Geometry: final body of the model. Coordinates: model frame, mm. A direction names the side the tool comes from. Give positions to 0.01 mm unless a question says otherwise; leave off trailing zeros. Write each loop counter-clockwise with the first axis right and the second up, starting at its lowest first coordinate (ties: lowest second). Pieces come first, ordered by that corner, then holes.
from build123d import *

# Parameters (mm, degrees)
BOSS_EXTRUDE1_DEPTH      = 280
BOSS_EXTRUDE1_DEPTH_BACK = 20


with BuildPart() as part:
    # Sketch1 → Boss-Extrude1 (new, two sides: drawn at the far end of the back side and taken through both)
    with BuildSketch(Plane.XY.offset(-BOSS_EXTRUDE1_DEPTH_BACK)):
        with BuildLine():
            Line((-170.37773053, -331.05), (-168.636, -331.05))
            Line((-168.636, -331.05), (-168.636, -59.198829312))
            ThreePointArc((-168.636, -59.198829312), (-165.748851618, -48.847485946), (-157.920969051, -41.484729004))
            Line((-157.920969051, -41.484729004), (-156.629100836, -40.807587282))
            Line((-156.629100836, -40.807587282), (-21.840950481, 29.842560493))
            Line((-21.840950481, 29.842560493), (4.633492495, 43.719324167))
            Line((4.633492495, 43.719324167), (3.240747138, 46.376439213))
            Line((3.240747138, 46.376439213), (-160.920969051, -39.670067673))
            ThreePointArc((-160.920969051, -39.670067673), (-168.748851618, -47.032824615), (-171.636, -57.384167981))
            Line((-171.636, -57.384167981), (-171.636, -331.05))
            Line((-171.636, -331.05), (-170.37773053, -331.05))
        make_face()
    extrude(amount=BOSS_EXTRUDE1_DEPTH + BOSS_EXTRUDE1_DEPTH_BACK)


solid = part.part
Q1. Pin query (flat end, axial travel): P1, Ø12, axis at y = -43, z = 241.5, coming from the -X side; P2, Ø6, axis at x = -125.5, z = 30, coming from the +Y side; P3, Ø5, axis at x = -61, z = 28.5, coming from the +Y side; P4, Ø4, axis at x = -88, y = -9, coming from the +Z side. Return the tip coordinate at first contact, or that it passes through.
Filled sheet:
P1: stops at x = -169.79
P2: stops at y = -19.53
P3: stops at y = 14.01
P4: passes through
Q2. Access query for faces 1 (the flat face through (-169, -141, -20)), 2 (the flat face through (-168.636, -197, 128)). Directions: +Z, -Z, +X, -X, +Y, -Y. A direction counts if a zero-diameter tool reaches every point of the face in a straight line with its end or side. Return the directions, or none.
Filled sheet:
face 1: -Z, +X, -X, +Y, -Y
face 2: +Z, -Z, +X, -Y
Q3. Section B-B on y = -223. Output: boundary loops of the cut face in (x, z).
Filled sheet:
outline: (-171.64, -20) - (-168.64, -20) - (-168.64, 280) - (-171.64, 280) - close
Q4. Ray query, line 1 along X through (y, z) = (-304, 180); line 2 along Y through (x, z) = (-51.5, 118); line 3 along Y through (x, z) = (-99, 52). Return the intervals inside material, ascending.
Filled sheet:
line 1: x = -171.64 to -168.64
line 2: y = 14.3 to 17.68
line 3: y = -10.6 to -7.21
Q5. Section C-C on x = -29. Output: boundary loops of the cut face in (y, z), plus the area to 3 significant figures.
Filled sheet:
outline: (26.09, -20) - (29.48, -20) - (29.48, 280) - (26.09, 280) - close
area: 1,020 mm2
Q6. Section A-A on z = 201. Output: boundary loops of the cut face in (x, y).
Filled sheet:
outline: (-171.64, -331.05) - (-168.64, -331.05) - (-168.64, -59.2) arc R20 cw to (-157.92, -41.48) - (4.63, 43.72) - (3.24, 46.38) - (-160.92, -39.67) arc R20 ccw to (-171.64, -57.38) - close
